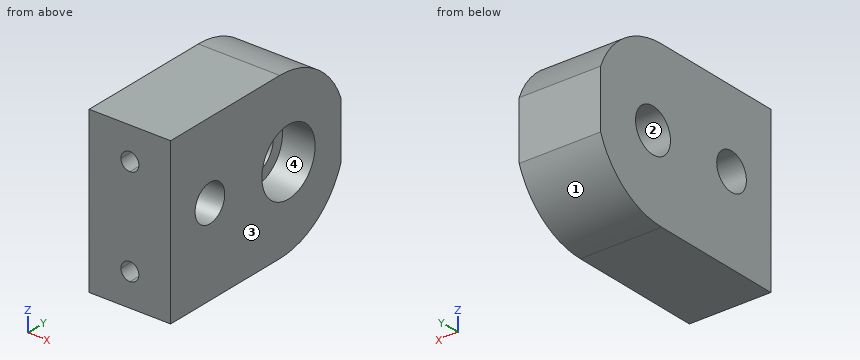
```python
from build123d import *

# Parameters (mm, degrees)
SKETCH_1_W               = 15
SKETCH_1_H               = 30
EXTRUDE_1_DEPTH          = 25
SKETCH_3_R               = 15
EXTRUDE_3_DEPTH          = 15
CUT_EXTRUDE_2_DEPTH      = 10
SKETCH_9_R               = 6.1
CUT_EXTRUDE_3_DEPTH      = 6
SKETCH_10_R              = 4
CUT_EXTRUDE_4_DEPTH      = 51.803543184
CUT_EXTRUDE_6_DEPTH      = 53.201532545
CUT_EXTRUDE_6_DEPTH_BACK = 53.201532545
SKETCH_5_R               = 3.4
CUT_EXTRUDE_8_DEPTH      = 52.439284598


with BuildPart() as part:
    # 草图1 → 凸台-拉伸1 (new body)
    with BuildSketch(Plane(origin=(0, 0, 0), x_dir=(1, 0, 0), z_dir=(0, 1, 0))):
        with Locations((7.5, -15)):
            Rectangle(SKETCH_1_W, SKETCH_1_H)
    extrude(amount=EXTRUDE_1_DEPTH)

    # 草图3 → 凸台-拉伸3 (add)
    with BuildSketch(Plane.ZY):
        with Locations((15, 25)):
            Circle(SKETCH_3_R)
    extrude(amount=-EXTRUDE_3_DEPTH)

    # 草图4 → 切除-拉伸2 (cut)
    with BuildSketch(Plane.XZ):
        with BuildLine():
            ThreePointArc((9.15, 24), (8.666726189, 25.166726189), (7.5, 25.65))
            Line((7.5, 25.65), (7.5, 22.35))
            ThreePointArc((7.5, 22.35), (8.666726189, 22.833273811), (9.15, 24))
        make_face()
        with BuildLine():
            Line((7.5, 22.35), (7.5, 25.65))
            ThreePointArc((7.5, 25.65), (5.85, 24), (7.5, 22.35))
        make_face()
        with BuildLine():
            ThreePointArc((9.15, 6), (8.666726189, 7.166726189), (7.5, 7.65))
            Line((7.5, 7.65), (7.5, 4.35))
            ThreePointArc((7.5, 4.35), (8.666726189, 4.833273811), (9.15, 6))
        make_face()
        with BuildLine():
            Line((7.5, 4.35), (7.5, 7.65))
            ThreePointArc((7.5, 7.65), (5.85, 6), (7.5, 4.35))
        make_face()
    extrude(amount=-CUT_EXTRUDE_2_DEPTH, mode=Mode.SUBTRACT)

    # 草图9 → 切除-拉伸3 (cut)
    with BuildSketch(Plane.ZY):
        with Locations((15, 27)):
            Circle(SKETCH_9_R)
    extrude(amount=-CUT_EXTRUDE_3_DEPTH, mode=Mode.SUBTRACT)

    # 草图10 → 切除-拉伸4 (cut, through all)
    with BuildSketch(Plane.ZY.offset(-6)):
        with Locations((15, 27)):
            Circle(SKETCH_10_R)
    extrude(amount=-CUT_EXTRUDE_4_DEPTH, mode=Mode.SUBTRACT)


with BuildPart() as body_2:
    # 镜向1: mirrored copy
    add(part.part.mirror(Plane(origin=(0, 0, 0), x_dir=(0, 0, 1), z_dir=(1, 0, 0))))

    # 草图12 → 切除-拉伸6 (cut, two sides: drawn at the far end of the back side and taken through both)
    with BuildSketch(Plane(origin=(0, 0, 0), x_dir=(0, 0, -1), z_dir=(1, 0, 0)).offset(-CUT_EXTRUDE_6_DEPTH_BACK)):
        with BuildLine():
            ThreePointArc((-9.614835193, 39), (-15, 40), (-20.385164807, 39))
            Line((-20.385164807, 39), (-9.614835193, 39))
        make_face()
    extrude(amount=CUT_EXTRUDE_6_DEPTH + CUT_EXTRUDE_6_DEPTH_BACK, mode=Mode.SUBTRACT)

    # 草图5 → 切除-拉伸8 (cut, through all)
    with BuildSketch(Plane.ZY):
        with Locations((15.95, 9)):
            Circle(SKETCH_5_R)
    extrude(amount=CUT_EXTRUDE_8_DEPTH, mode=Mode.SUBTRACT)


solid = body_2.part
```
Work out the finished part from the listing and answer in its coordinate system (mm). Face numbers are marked on the shaded views. Give positions to 0.01 mm unless a question says otherwise; leave off trailing zeros. Loops run counter-clockwise (first coordinate to the right, second up) from the corner with the lowest first, then second, coordinate; pieces in that order, holes last. Notation, with made-up numbers: (-28, 84) -> (-6, 84) arc R19 ccw to (-6, 104) -> close; hole circle Ø3 at (23, 64). An arc over 180 degrees is marked (long way). Put each result on its own line as item: value. Start each with the question number.
Item 1: Find the intervals of material crossed by L1, parallel to Z at x = -3.5, y = 9; L2, parallel to Y at x = -8, z = 15; L3, parallel to Y at x = -2.6, z = 15, in increasing order. Write a range as [from, to].
Item 2: The mould has two halves that part along Z. Classify the marked faces 1, 2, 3 and 4: released by +Z, released by -Z, zero draft, split by the parting line, or undercut.
Item 3: The part is cut by section B-B (x = -13). Give the vertices of the cut face in (y, z).
Item 4: The part is cut by section C-C (z = 15.95). Give the vertices of the cut face in (x, y).
Item 5: The part is cut by section D-D (y = 24.5). Give the vertices of the cut face in (x, z), then the cut area to 3 significant figures.
Item 6: The part is cut by section A-A (y = 9). Give the vertices of the cut face in (x, z).
Item 7: Each of these flat-tipped pins is pushed along its axis until it touches: P1, Ø10.5, axis at y = 27, z = 15, coming from the -X side; P2, Ø2.5, axis at x = -7.5, z = 6, coming from the -Y side; P3, Ø3, axis at x = -9, y = 28.5, coming from the +Z side. Where does it stop, or does it pass through?
Answers below:
1. L1: [0, 12.55], [19.35, 30]
1. L2: [0, 5.74], [12.26, 23], [31, 39]
1. L3: [0, 5.74], [12.26, 20.9], [33.1, 39]
2. face 1: released by -Z
2. face 2: undercut
2. face 3: zero draft
2. face 4: undercut
3. outline: (0, 0) -> (25, 0) arc R15 ccw to (39, 9.61) -> (39, 20.39) arc R15 ccw to (25, 30) -> (0, 30) -> close; hole circle Ø6.8 at (9, 15.95); hole circle Ø8 at (27, 15)
4. outline: (-15, 0) -> (0, 0) -> (0, 5.6) -> (-15, 5.6) -> close; (-15, 12.4) -> (0, 12.4) -> (0, 20.97) -> (-6, 20.97) -> (-6, 23.11) -> (-15, 23.11) -> close; (-15, 30.89) -> (-6, 30.89) -> (-6, 33.03) -> (0, 33.03) -> (0, 39) -> (-15, 39) -> close
5. outline: (-15, 0) -> (0, 0) -> (0, 9.44) -> (-6, 9.44) -> (-6, 11.88) -> (-15, 11.88) -> close; (-15, 18.12) -> (-6, 18.12) -> (-6, 20.56) -> (0, 20.56) -> (0, 30) -> (-15, 30) -> close
5. area: 327 mm2
6. outline: (-15, 0) -> (0, 0) -> (0, 12.55) -> (-15, 12.55) -> close; (-15, 19.35) -> (0, 19.35) -> (0, 30) -> (-15, 30) -> close; hole circle Ø3.3 at (-7.5, 6); hole circle Ø3.3 at (-7.5, 24)
7. P1: x = -15
7. P2: y = 10
7. P3: z = 29.87
